Work out the finished part from the listing and answer in its coordinate system (mm). A direction names the side the tool comes from. Give positions to 0.01 mm unless a question says otherwise; leave off trailing zeros. Loops run counter-clockwise (first coordinate to the right, second up) from the corner with the lowest first, then second, coordinate; pieces in that order, holes last. Notation, with made-up numbers: (-16, 88) -> (11, 88) arc R9 ccw to (11, 93) -> close; hole circle Ø6 at (85.5, 51.5). An arc over 180 degrees is marked (long way). Answer as CSV lines item,"result". Start each with the question number.
1. Find the intervals of material crossed by line 1 along Y through (x, z) = (-0.9, 0.5); line 2 along X through (y, z) = (2, -0.25); line 3 along Z through (x, y) = (0.1, -2.2), in increasing order.
2. Find section A-A, the plane x = 0. Give the vertices of the cut face in (y, z), and give its area (3 significant figures).
3. Find section D-D, the plane x = 2.15. Give the vertices of the cut face in (y, z), and give its area (3 significant figures).
4. Find section C-C, the plane x = -2. Give the vertices of the cut face in (y, z).
5. A tool of negligible diameter and unlimited length cuts with its end or side. For faces 1 (the face through (0.54, -2.44, -2.46)), 2 (the face through (0, -2, 0)), from which of +Z, -Z, +X, -X, +Y, -Y can it reach the whole face along a straight path? Write none if from no direction.
from build123d import *

# Parameters (mm, degrees)
SKETCH1_R           = 1.5
BOSS_EXTRUDE1_DEPTH = 7
SKETCH2_R           = 2.5
BOSS_EXTRUDE2_DEPTH = 5
FILLET2_R           = 0.3


with BuildPart() as part:
    # Sketch1 → Boss-Extrude1 (new body)
    with BuildSketch(Plane.XY):
        Circle(SKETCH1_R)
    extrude(amount=BOSS_EXTRUDE1_DEPTH)

    # Sketch2 → Boss-Extrude2 (add)
    with BuildSketch(Plane(origin=(0, 0, 0), x_dir=(-1, 0, 0), z_dir=(0, 0, -1))):
        Circle(SKETCH2_R)
    extrude(amount=BOSS_EXTRUDE2_DEPTH)

    # Fillet2
    fillet2_edges = [part.edges().sort_by_distance(p)[0] for p in [
        (-1.5, 0, 7),
    ]]
    fillet(fillet2_edges, radius=FILLET2_R)


solid = part.part
Resolved:
1,line 1,"y = -1.2 to 1.2"
1,line 2,"x = -1.5 to 1.5"
1,line 3,"z = -5 to 0"
2,outline,"(-2.5, -5) -> (2.5, -5) -> (2.5, 0) -> (1.5, 0) -> (1.5, 6.7) arc R0.3 ccw to (1.2, 7) -> (-1.2, 7) arc R0.3 ccw to (-1.5, 6.7) -> (-1.5, 0) -> (-2.5, 0) -> close"
2,area,"46.0 mm^2"
3,outline,"(-1.28, -5) -> (1.28, -5) -> (1.28, 0) -> (-1.28, 0) -> close"
3,area,"12.8 mm^2"
4,outline,"(-1.5, -5) -> (1.5, -5) -> (1.5, 0) -> (-1.5, 0) -> close"
5,face 1,"+Z, -Z"
5,face 2,"+Z"
